```python
from build123d import *

# Parameters (mm, degrees)
SKETCH_1_R            = 23
EXTRUDE_1_DEPTH       = 5
SKETCH_2_R            = 1.6
CUT_EXTRUDE_1_DEPTH   = 33.908965344
SKETCH_3_R            = 1
CUT_EXTRUDE_2_DEPTH   = 33.908965344
SKETCH_4_W            = 14.5
SKETCH_4_H            = 1
SKETCH_5_R            = 2.1
CUT_EXTRUDE_3_DEPTH   = 33.771939229
SKETCH_6_R            = 3.5
SKETCH_6_R_2          = 2.5
CUT_EXTRUDE_1_2_DEPTH = 2
SKETCH_7_R            = 3.5
CUT_EXTRUDE_4_DEPTH   = 1
CHAMFER_1_SIZE        = 0.5


with BuildPart() as part:
    # 草图1 → 凸台-拉伸1 (new body)
    with BuildSketch(Plane(origin=(0, 0, 0), x_dir=(1, 0, 0), z_dir=(0, 1, 0))):
        with Locations(Location((0, 0, 0), (0, 0, 270))):
            Circle(SKETCH_1_R)
    extrude(amount=EXTRUDE_1_DEPTH)

    # 草图2 → Cut-Extrude 1 (cut, through all)
    with BuildSketch(Plane(origin=(0, 5, 0), x_dir=(1, 0, 0), z_dir=(0, 1, 0))):
        with Locations(Location((0, 20, 0), (0, 0, 270))):
            Circle(SKETCH_2_R)
        with Locations(Location((20.001, 0.001, 0), (0, 0, 270))):
            Circle(SKETCH_2_R)
        with Locations(Location((0.002, -20, 0), (0, 0, 270))):
            Circle(SKETCH_2_R)
        with Locations(Location((-19.999, -0.001, 0), (0, 0, 270))):
            Circle(SKETCH_2_R)
    extrude(amount=-CUT_EXTRUDE_1_DEPTH, mode=Mode.SUBTRACT)

    # 草图3 → 切除-拉伸2 (cut, through all)
    with BuildSketch(Plane(origin=(0, 5, 0), x_dir=(1, 0, 0), z_dir=(0, 1, 0))):
        with Locations(Location((14.142135624, 14.142135624, 0), (0, 0, 270))):
            Circle(SKETCH_3_R)
        with Locations(Location((14.142135624, -14.142135624, 0), (0, 0, 270))):
            Circle(SKETCH_3_R)
        with Locations(Location((-14.142135624, -14.142135624, 0), (0, 0, 270))):
            Circle(SKETCH_3_R)
        with Locations(Location((-14.142135624, 14.142135624, 0), (0, 0, 270))):
            Circle(SKETCH_3_R)
    extrude(amount=-CUT_EXTRUDE_2_DEPTH, mode=Mode.SUBTRACT)

    # 草图4 → 切除-旋转1 (revolve, cut)
    with BuildSketch(Plane.XY, mode=Mode.PRIVATE) as cut_revolve_1_sk:
        with Locations((7.25, 4.5)):
            Rectangle(SKETCH_4_W, SKETCH_4_H)
        Polygon((18.5, 1.5), (18.5, 5), (14.5, 5), (14.5, 4), align=None)
    revolve(cut_revolve_1_sk.sketch.rotate(Axis((0, 0, 0), (0, 1, 0)), 90), axis=Axis((0, 0, 0), (0, 1, 0)), mode=Mode.SUBTRACT)

    # 草图5 → 切除-拉伸3 (cut, through all)
    with BuildSketch(Plane(origin=(0, 4, 0), x_dir=(1, 0, 0), z_dir=(0, 1, 0))):
        with Locations(Location((4.242640687, -4.242640687, 0), (0, 0, 270))):
            Circle(SKETCH_5_R)
    extrude(amount=-CUT_EXTRUDE_3_DEPTH, mode=Mode.SUBTRACT)

    # 草图6 → Cut-Extrude 1 2 (cut)
    with BuildSketch(Plane(origin=(0, 4, 0), x_dir=(1, 0, 0), z_dir=(0, 1, 0))):
        with Locations((4.242640687, -4.242640687)):
            Circle(SKETCH_6_R)
        with Locations((4.242640687, -4.242640687)):
            Circle(SKETCH_6_R_2, mode=Mode.SUBTRACT)
    extrude(amount=-CUT_EXTRUDE_1_2_DEPTH, mode=Mode.SUBTRACT)

    # 草图7 → 切除-拉伸4 (cut)
    with BuildSketch(Plane(origin=(0, 4, 0), x_dir=(1, 0, 0), z_dir=(0, 1, 0))):
        with Locations((4.242640687, -4.242640687)):
            Circle(SKETCH_7_R)
    extrude(amount=-CUT_EXTRUDE_4_DEPTH, mode=Mode.SUBTRACT)

    # 倒角1
    chamfer_1_edges = [part.edges().sort_by_distance(p)[0] for p in [
        (0, 5, -21.6),
        (21.307215325, 5, -0.925013812),
        (1.578782453, 5, 20.271582579),
        (-21.306855112, 5, -0.920691384),
    ]]
    chamfer(chamfer_1_edges, length=CHAMFER_1_SIZE)


solid = part.part
```
The listing builds one solid part. Answer for the finished solid, in the listing's coordinates (mm). A direction names the side the tool comes from. Give positions to 0.01 mm unless a question says otherwise; leave off trailing zeros. Order: outer loops, then holes, each group sorted by start corner. A loop starts at its lowest first (then second) coordinate and runs counter-clockwise, first axis right, second up. Notation, with made-up numbers: (27, 32.25) - (40, 32.25) arc R21 ccw to (40, 41.25) - close; hole circle Ø7 at (25, 33). An arc over 180 degrees is marked (long way). Answer in a Markdown table with one row per item. Add a question column.
Q1. The part is cut by section B-B (y = 0.9). Give the number of separate pieces and of enclosed holes in the cut face, then the cut area to 3 significant figures.
Q2. The part is cut by section A-A (z = 20). Determine the outline of the cut face in (x, y), then the cut area to 3 significant figures.
Q3. For a pull along Z with two mould halves and no side action, classify faces 1 (the cylindrical face through (19.394, 2.465, 12.365)), 2 (the flat face through (0, 0, 0)), 3 (the conical face through (-0.066, 4.635, 21.734)), 4 (the cylindrical face through (0.483, 2.282, 21.526)) as released by +Z, released by -Z, zero draft, split by the parting line, or undercut.
Q4. Given P1, Ø3, axis at x = 7.5, y = 2.5, coming from the -Z side; P2, Ø3.5, axis at x = 0, z = -20, coming from the +Y side; P3, Ø2.5, axis at x = -14.14, z = 14.14, coming from the -Y side; P4, Ø2, axis at x = -3.5, y = 3.5, coming from the +Z side, each flat-ended and moving along its own axis, determine where each tip first touches the part or whether it passes through.
Q5. Find the intervals of material crossed by line 1 along Z through (x, y) = (12, 1.6); line 2 along Z through (x, y) = (-3, 2.1); line 3 along X through (y, z) = (2.9, 3.5), in increasing order. Write a range as [from, to].
Q6. Which of the six approach directions +Z, -Z, +X, -X, +Y, -Y give full straight-line access (tool end or side, diameter ignored) to faces 5 (the flat face through (6, 2, 7)), 6 (the cylindrical face through (-14.098, 2.535, 13.143))?
Determined:
| question | item | result |
|---|---|---|
| 1 | separate pieces | 1 |
| 1 | enclosed holes | 9 |
| 1 | area | 1,600 mm² |
| 2 | outline | (-11.36, 0) - (-1.6, 0) - (-1.6, 4.5) - (-2.1, 5) - (-11.36, 5) - close; (1.6, 0) - (11.36, 0) - (11.36, 5) - (2.1, 5) - (1.6, 4.5) - close |
| 2 | area | 97.3 mm² |
| 3 | face 1 | split by the parting line |
| 3 | face 2 | zero draft |
| 3 | face 3 | undercut |
| 3 | face 4 | undercut |
| 4 | P1 | stops at z = -22.2 |
| 4 | P2 | stops at y = 4.65 |
| 4 | P3 | stops at y = 0 |
| 4 | P4 | stops at z = 22.86 |
| 5 | line 1 | z = [-19.62, -14.08], [-13.87, 13.87], [14.08, 19.62] |
| 5 | line 2 | z = [-22.8, -18.26], [-17.28, 17.28], [18.26, 22.8] |
| 5 | line 3 | x = [-22.73, -18.17], [-15.88, 0.82], [1.86, 2.28], [6.21, 6.63], [7.66, 15.88], [18.17, 22.73] |
| 6 | face 5 | +Y |
| 6 | face 6 | +Y, -Y |
